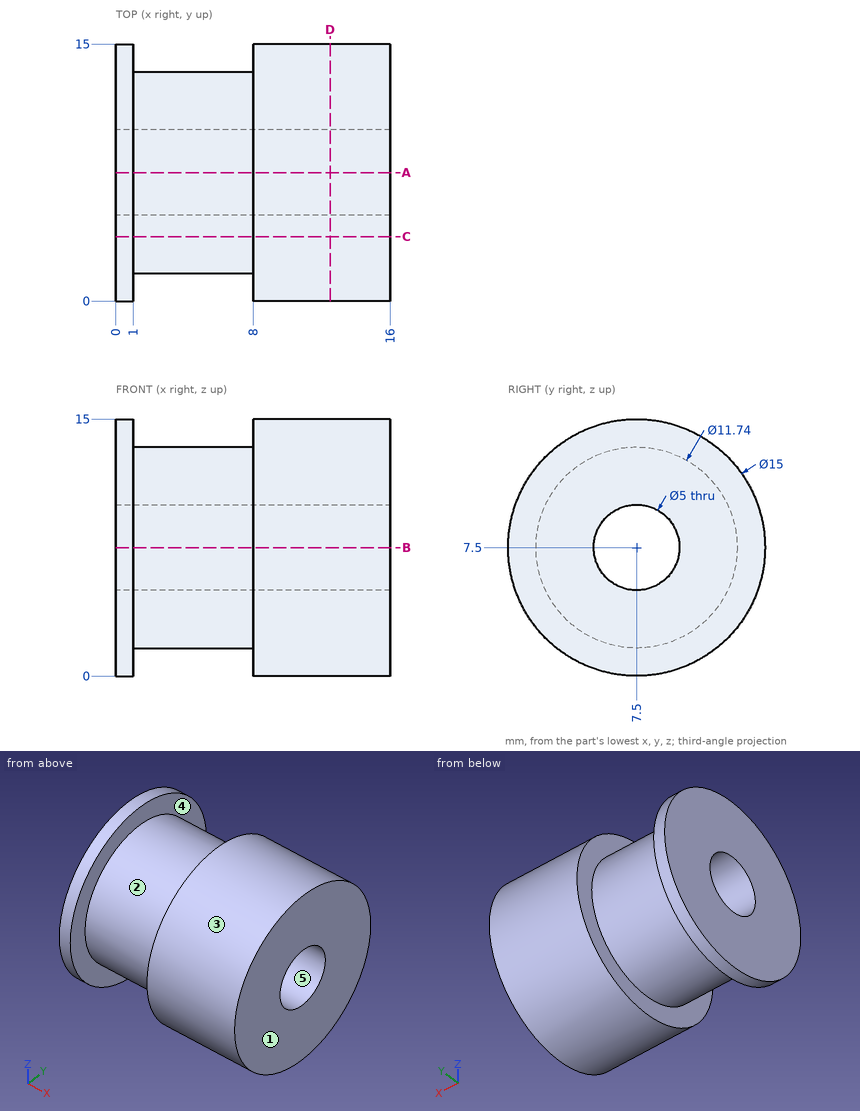
Geometry: see drawing. Coordinates: mm, zero at the bounding-box minimum. A direction names the side the tool comes from. Round coordinates to 2 decimals unless told otherwise and drop trailing zeros. Write each loop counter-clockwise with the first axis right and the second up, starting at its lowest first coordinate (ties: lowest second). Pieces come first, ordered by that corner, then holes. Notation, with made-up numbers: (80.5, 55) - (109.5, 55) arc R32 cw to (109.5, 94) - close; hole circle Ø8 at (45.25, 18). An arc over 180 degrees is marked (long way). Use CSV: the item, a comma, the result in double quotes. Start each with the question number.
(1) First-contact query: pin 1 Ø4 at (x, y) = (9.5, 10.5) entering from +Z; pin 2 Ø2 at (x, y) = (4.5, 2.5) entering from -Z; pin 3 Ø1.5 at (x, y) = (9, 8.5) entering from +Z. Flat tips, straight axial feed; report the tip coordinate or a pass-through.
(2) Cut plane A-A, the plane y = 7.5. Return loops of the section in (x, z).
(3) Cut plane D-D, the plane x = 12.5. Return loops of the section in (y, z), and give its area (3 significant figures).
(4) Material intervals for probe 1 along X at (y, z) = (10.5, 0.75); probe 2 along Y at (x, z) = (7.5, 7.5); probe 3 along Y at (x, z) = (9.25, 8.25), sorted ascending. Write a range as [from, to].
(5) Set-up query: the marked faces 1 and 2. Return all of +Z, -Z, +X, -X, +Y, -Y with unobstructed straight access to the full face (end or side cutting, diameter ignored); none if empty.
(6) Mould query, pull axis Y, two halves, no side actions, for the marked faces 3, 4 and 5. Classes: pulls with the +Y half, pulls with the -Y half, needs draft (parallel to the pull), parting line crosses it, or undercut.
(7) Cut plane C-C, the plane y = 3.75. Return loops of the section in (x, z), and give its area (3 significant figures).
Geometry says:
1,pin 1,"z = 14.93"
1,pin 2,"z = 3.2"
1,pin 3,"z = 15"
2,outline,"(0, 0) - (1, 0) - (1, 1.63) - (8, 1.63) - (8, 0) - (16, 0) - (16, 5) - (0, 5) - close; (0, 10) - (16, 10) - (16, 15) - (8, 15) - (8, 13.37) - (1, 13.37) - (1, 15) - (0, 15) - close"
3,outline,"circle Ø15 at (7.5, 7.5); hole circle Ø5 at (7.5, 7.5)"
3,area,"157 mm²"
4,probe 1,"[0, 1], [8, 16]"
4,probe 2,"[1.63, 5], [10, 13.37]"
4,probe 3,"[0.04, 5.12], [9.88, 14.96]"
5,face 1,"+Z, -Z, +X, +Y, -Y"
5,face 2,"none"
6,face 3,"parting line crosses it"
6,face 4,"needs draft"
6,face 5,"undercut"
7,outline,"(0, 1) - (1, 1) - (1, 2.98) - (8, 2.98) - (8, 1) - (16, 1) - (16, 14) - (8, 14) - (8, 12.02) - (1, 12.02) - (1, 14) - (0, 14) - close"
7,area,"180 mm²"
